Design review of the part built by this model. Coordinates are the model's own, in mm. A direction names the side the tool comes from. Coordinates: 2 decimals unless noted, no trailing zeros. Loops run counter-clockwise (first coordinate to the right, second up) from the corner with the lowest first, then second, coordinate; pieces in that order, holes last. Notation, with made-up numbers: M 43.25,59.5 L 97.25,59.5 A19 cw 97.25,71.5 Z; hole C 13.25,7.25 d1. An arc over 180 degrees is marked long. Write item = value, one per line. Start each with the question number.
from build123d import *

# Parameters (mm, degrees)
SKETCH1_W                = 50
SKETCH1_H                = 25
SKETCH1_R                = 1.3
SKETCH1_R_2              = 4.5
BOSS_EXTRUDE1_DEPTH      = 2.5
SKETCH2_W                = 50
SKETCH2_H                = 12
BOSS_EXTRUDE2_DEPTH      = 3
SKETCH3_W                = 50
SKETCH3_H                = 28
BOSS_EXTRUDE3_DEPTH      = 3
SKETCH4_R                = 1.3
CUT_EXTRUDE1_DEPTH       = 16
SKETCH5_W                = 53
SKETCH5_H                = 32.5
SKETCH5_R                = 1.6
SKETCH5_W_2              = 42
SKETCH5_H_2              = 21.5
BOSS_EXTRUDE4_DEPTH      = 4
SKETCH7_R                = 8
CUT_EXTRUDE2_DEPTH       = 5
SKETCH8_W                = 24.55
SKETCH8_H                = 21.5
CUT_EXTRUDE3_DEPTH       = 3.8
BOSS_EXTRUDE6_DEPTH      = 22.95
BOSS_EXTRUDE7_DEPTH      = 2
SKETCH11_R               = 1.6
CUT_EXTRUDE4_DEPTH       = 1.2
SKETCH12_W               = 7
SKETCH12_H               = 21
SKETCH12_R               = 1.6
BOSS_EXTRUDE8_DEPTH      = 7.8
SKETCH13_W               = 0.7
SKETCH13_H               = 5
SKETCH13_H_2             = 4
CUT_EXTRUDE5_DEPTH       = 51
CUT_EXTRUDE5_DEPTH_BACK  = 25.95
SKETCH14_W               = 28
SKETCH14_H               = 10
CUT_EXTRUDE6_DEPTH       = 1
CUT_EXTRUDE6_DEPTH_BACK  = 75.95
SKETCH16_R               = 3
CUT_EXTRUDE8_DEPTH       = 3
SKETCH15_R               = 1.6
CUT_EXTRUDE9_DEPTH       = 5
SKETCH17_W               = 16.3
SKETCH17_H               = 5
CUT_EXTRUDE10_DEPTH      = 3.2
SKETCH18_R               = 1.45
CUT_EXTRUDE11_DEPTH      = 5
SKETCH19_R               = 1.6
CUT_EXTRUDE12_DEPTH      = 1.0000001
CUT_EXTRUDE12_DEPTH_BACK = 10
SKETCH20_W               = 17.95
SKETCH20_H               = 5
CUT_EXTRUDE14_DEPTH      = 1
CUT_EXTRUDE14_DEPTH_BACK = 32.8
SKETCH21_W               = 16.3
SKETCH21_H               = 5
SKETCH21_R               = 1.45
BOSS_EXTRUDE11_DEPTH     = 2
SKETCH22_W               = 55
SKETCH22_H               = 5
BOSS_EXTRUDE12_DEPTH     = 25
SKETCH23_R               = 10.5
BOSS_EXTRUDE13_DEPTH     = 2
SKETCH24_R               = 1.3
SKETCH24_R_2             = 0.75
CUT_EXTRUDE16_DEPTH      = 7
SKETCH25_R               = 2.5
SKETCH25_R_2             = 1.3
CUT_EXTRUDE17_DEPTH      = 4


with BuildPart() as part:
    # Sketch1 → Boss-Extrude1 (new body, symmetric)
    with BuildSketch(Plane(origin=(0, 0, 0), x_dir=(1, 0, 0), z_dir=(0, 1, 0))):
        Rectangle(SKETCH1_W, SKETCH1_H)
        with Locations((-11.25, 0)):
            Circle(SKETCH1_R, mode=Mode.SUBTRACT)
        with Locations((11.25, 0)):
            Circle(SKETCH1_R_2, mode=Mode.SUBTRACT)
    extrude(amount=BOSS_EXTRUDE1_DEPTH, both=True)

    # Sketch2 → Boss-Extrude2 (add)
    with BuildSketch(Plane.XY.offset(12.5)):
        with Locations((0, 3.5)):
            Rectangle(SKETCH2_W, SKETCH2_H)
    extrude(amount=BOSS_EXTRUDE2_DEPTH)

    # Sketch3 → Boss-Extrude3 (add)
    with BuildSketch(Plane(origin=(0, 9.5, 0), x_dir=(1, 0, 0), z_dir=(0, 1, 0))):
        with Locations((0, -1.5)):
            Rectangle(SKETCH3_W, SKETCH3_H)
    extrude(amount=BOSS_EXTRUDE3_DEPTH)

    # Sketch4 → Cut-Extrude1 (cut, through all)
    with BuildSketch(Plane(origin=(0, 12.5, 0), x_dir=(1, 0, 0), z_dir=(0, 1, 0))):
        with Locations((11.25, 0)):
            Circle(SKETCH4_R)
        with Locations((-11.25, 0)):
            Circle(SKETCH4_R)
    extrude(amount=-CUT_EXTRUDE1_DEPTH, mode=Mode.SUBTRACT)

    # Sketch5 → Boss-Extrude4 (add)
    with BuildSketch(Plane.XZ.offset(2.5)):
        with Locations((21.45, -0.05)):
            Rectangle(SKETCH5_W, SKETCH5_H)
        with Locations((45.75, -5)):
            Circle(SKETCH5_R, mode=Mode.SUBTRACT)
        with Locations((45.75, 4.9)):
            Circle(SKETCH5_R, mode=Mode.SUBTRACT)
        with Locations((-2.85, 4.9)):
            Circle(SKETCH5_R, mode=Mode.SUBTRACT)
        with Locations((-2.85, -5)):
            Circle(SKETCH5_R, mode=Mode.SUBTRACT)
        with Locations((21.45, -0.05)):
            Rectangle(SKETCH5_W_2, SKETCH5_H_2, mode=Mode.SUBTRACT)
    extrude(amount=BOSS_EXTRUDE4_DEPTH)

    # Sketch7 → Cut-Extrude2 (cut)
    with BuildSketch(Plane.XZ.offset(2.5)):
        with Locations((11.25, 0)):
            Circle(SKETCH7_R)
    extrude(amount=-CUT_EXTRUDE2_DEPTH, mode=Mode.SUBTRACT)

    # Sketch8 → Cut-Extrude3 (cut)
    with BuildSketch(Plane.XZ.offset(2.5)):
        with Locations((12.725, -0.05)):
            Rectangle(SKETCH8_W, SKETCH8_H)
    extrude(amount=-CUT_EXTRUDE3_DEPTH, mode=Mode.SUBTRACT)

    # Sketch9 → Boss-Extrude6 (add)
    with BuildSketch(Plane(origin=(25, 0, 0), x_dir=(0, 0, -1), z_dir=(1, 0, 0))):
        Polygon((12.5, 2.5), (-16.2, 2.5), (-16.2, -2.5), (-10.7, -2.5), (-10.7, 1.3), (10.8, 1.3), (10.8, -2.5), (12.5, -2.5), align=None)
    extrude(amount=BOSS_EXTRUDE6_DEPTH)

    # Sketch10 → Boss-Extrude7 (add)
    with BuildSketch(Plane(origin=(47.95, 0, 0), x_dir=(0, 0, -1), z_dir=(1, 0, 0))):
        Polygon((16.3, -2.5), (12.5, -2.5), (12.5, 2.5), (-16.2, 2.5), (-16.2, -6.5), (16.3, -6.5), align=None)
    extrude(amount=BOSS_EXTRUDE7_DEPTH)

    # Sketch11 → Cut-Extrude4 (cut)
    with BuildSketch(Plane.XZ.offset(-1.3)):
        with Locations((-2.85, 4.9)):
            Circle(SKETCH11_R)
        with Locations((-2.85, -5)):
            Circle(SKETCH11_R)
        with Locations((45.75, 4.9)):
            Circle(SKETCH11_R)
        with Locations((45.75, -5)):
            Circle(SKETCH11_R)
    extrude(amount=-CUT_EXTRUDE4_DEPTH, mode=Mode.SUBTRACT)

    # Sketch12 → Boss-Extrude8 (add)
    with BuildSketch(Plane.XZ.offset(-1.3)):
        with Locations((46.45, 0.2)):
            Rectangle(SKETCH12_W, SKETCH12_H)
        with Locations((45.75, 4.9)):
            Circle(SKETCH12_R, mode=Mode.SUBTRACT)
        with Locations((45.75, -5)):
            Circle(SKETCH12_R, mode=Mode.SUBTRACT)
    extrude(amount=BOSS_EXTRUDE8_DEPTH)

    # Sketch13 → Cut-Extrude5 (cut, two sides)
    with BuildSketch(Plane.ZY.offset(-25)) as cut_extrude5_sk:
        with Locations((15.85, 0)):
            Rectangle(SKETCH13_W, SKETCH13_H)
        with Locations((15.85, -4.5)):
            Rectangle(SKETCH13_W, SKETCH13_H_2)
    extrude(amount=CUT_EXTRUDE5_DEPTH, mode=Mode.SUBTRACT)
    extrude(cut_extrude5_sk.sketch, amount=-CUT_EXTRUDE5_DEPTH_BACK, mode=Mode.SUBTRACT)

    # Sketch14 → Cut-Extrude6 (cut, two sides)
    with BuildSketch(Plane.ZY.offset(25)) as cut_extrude6_sk:
        with Locations((1.5, 7.5)):
            Rectangle(SKETCH14_W, SKETCH14_H)
    extrude(amount=CUT_EXTRUDE6_DEPTH, mode=Mode.SUBTRACT)
    extrude(cut_extrude6_sk.sketch, amount=-CUT_EXTRUDE6_DEPTH_BACK, mode=Mode.SUBTRACT)

    # Sketch16 → Cut-Extrude8 (cut)
    with BuildSketch(Plane(origin=(0, 2.5, 0), x_dir=(1, 0, 0), z_dir=(0, 1, 0))):
        with Locations((-2.85, 5)):
            Circle(SKETCH16_R)
        with Locations((-2.85, -4.9)):
            Circle(SKETCH16_R)
        with Locations((45.75, 5)):
            Circle(SKETCH16_R)
        with Locations((45.75, -4.9)):
            Circle(SKETCH16_R)
    extrude(amount=-CUT_EXTRUDE8_DEPTH, mode=Mode.SUBTRACT)

    # Sketch15 → Cut-Extrude9 (cut)
    with BuildSketch(Plane(origin=(0, 2.5, 0), x_dir=(1, 0, 0), z_dir=(0, 1, 0))):
        with Locations((-2.85, 5)):
            Circle(SKETCH15_R)
        with Locations((-2.85, -4.9)):
            Circle(SKETCH15_R)
    extrude(amount=-CUT_EXTRUDE9_DEPTH, mode=Mode.SUBTRACT)

    # Sketch17 → Cut-Extrude10 (cut)
    with BuildSketch(Plane.XY.offset(15.5)):
        with Locations((8.9, 0)):
            Rectangle(SKETCH17_W, SKETCH17_H)
        with Locations((31, 0)):
            Rectangle(SKETCH17_W, SKETCH17_H)
    extrude(amount=-CUT_EXTRUDE10_DEPTH, mode=Mode.SUBTRACT)

    # Sketch18 → Cut-Extrude11 (cut)
    with BuildSketch(Plane.XY.offset(12.3)):
        with Locations((8.95, 0)):
            Circle(SKETCH18_R)
        with Locations((30.95, 0)):
            Circle(SKETCH18_R)
    extrude(amount=-CUT_EXTRUDE11_DEPTH, mode=Mode.SUBTRACT)

    # Sketch19 → Cut-Extrude12 (cut, two sides)
    with BuildSketch(Plane(origin=(0, 2.5, 0), x_dir=(1, 0, 0), z_dir=(0, 1, 0))) as cut_extrude12_sk:
        with Locations((33.75, 0)):
            Circle(SKETCH19_R)
    extrude(amount=CUT_EXTRUDE12_DEPTH, mode=Mode.SUBTRACT)
    extrude(cut_extrude12_sk.sketch, amount=-CUT_EXTRUDE12_DEPTH_BACK, mode=Mode.SUBTRACT)

    # Sketch20 → Cut-Extrude14 (cut, two sides)
    with BuildSketch(Plane.XY.offset(15.5)) as cut_extrude14_sk:
        with Locations((-16.025, 0)):
            Rectangle(SKETCH20_W, SKETCH20_H)
    extrude(amount=CUT_EXTRUDE14_DEPTH, mode=Mode.SUBTRACT)
    extrude(cut_extrude14_sk.sketch, amount=-CUT_EXTRUDE14_DEPTH_BACK, mode=Mode.SUBTRACT)

    # Sketch21 → Boss-Extrude11 (add)
    with BuildSketch(Plane.XY.offset(15.5)):
        with Locations((8.9, 0)):
            Rectangle(SKETCH21_W, SKETCH21_H)
        with Locations((8.95, 0)):
            Circle(SKETCH21_R, mode=Mode.SUBTRACT)
        Polygon((0.75, -2.5), (0.75, 2.5), (-7.05, 2.5), (-7.05, -2.5), (-5.05, -2.5), (-5.05, -6.5), (49.95, -6.5), (49.95, 2.5), (39.15, 2.5), (39.15, -2.5), (22.85, -2.5), (22.85, 2.5), (17.05, 2.5), (17.05, -2.5), align=None)
        with Locations((31, 0)):
            Rectangle(SKETCH21_W, SKETCH21_H)
        with Locations((30.95, 0)):
            Circle(SKETCH21_R, mode=Mode.SUBTRACT)
    extrude(amount=BOSS_EXTRUDE11_DEPTH)

    # Sketch22 → Boss-Extrude12 (add)
    with BuildSketch(Plane.XZ.offset(6.5)):
        with Locations((22.45, 15)):
            Rectangle(SKETCH22_W, SKETCH22_H)
    extrude(amount=BOSS_EXTRUDE12_DEPTH)

    # Sketch23 → Boss-Extrude13 (add)
    with BuildSketch(Plane.XY.offset(17.5)):
        with Locations((22.45, -19.5)):
            Circle(SKETCH23_R)
    extrude(amount=BOSS_EXTRUDE13_DEPTH)

    # Sketch24 → Cut-Extrude16 (cut)
    with BuildSketch(Plane.XY.offset(19.5)):
        with Locations((22.45, -19.5)):
            Circle(SKETCH24_R)
        with Locations((22.45, -11.8)):
            Circle(SKETCH24_R_2)
        with Locations((22.45, -27.2)):
            Circle(SKETCH24_R_2)
    extrude(amount=-CUT_EXTRUDE16_DEPTH, mode=Mode.SUBTRACT)

    # Sketch25 → Cut-Extrude17 (cut)
    with BuildSketch(Plane(origin=(0, 0, 12.5), x_dir=(-1, 0, 0), z_dir=(0, 0, -1))):
        with Locations((-22.45, -19.5)):
            Circle(SKETCH25_R)
        with Locations((-22.45, -19.5)):
            Circle(SKETCH25_R_2, mode=Mode.SUBTRACT)
    extrude(amount=-CUT_EXTRUDE17_DEPTH, mode=Mode.SUBTRACT)


solid = part.part
Q1. For faces 5 (the face through (31, -2.5, 14)), 6 (the face through (22, -2.5, -14)), 7 (the face through (11.96, -19.04, 18.49)), 8 (the face through (22, -16, 12.5)), 9 (the face through (21, -21, 16.5)), list the 3-axis set-ups (+Z, -Z, +X, -X, +Y, -Y) from which the entire face can be reached by the end or side of a thin tool; tool diameter is ignored.
Q2. Add section B-B on z = 0. State the section outline as (x, y) points.
Q3. Add section C-C on x = -2.85. State the section outline as (y, z) points.
Q4. To check wall thickness, follow line 1 (X direction, y = 1.65, z = 0); line 2 (Z direction, x = -2.85, y = 1.1); line 3 (Z direction, x = -2.85, y = -4.7). State the ranges of each line that lie inside material, in increasing order. Write a range as from..to.
Q5. Mouldability with a two-part tool opening along Z and no side actions: class faces 1 (the face through (44.57, -3.46, -3.92)), 2 (the face through (24, 1.3, 0)), 3 (the face through (10, -1, 16)), 4 (the face through (22, -5, -16.3)) as released by +Z, released by -Z, zero draft, split by the parting line, or undercut.
Q6. Clearance check with flat-ended pins moving along their axes: P1, Ø1.7, axis at x = 45.5, z = 6, coming from the +Y side; P2, Ø7.5, axis at x = 17.5, y = -24.5, coming from the -Z side; P3, Ø3, axis at x = 17, z = -14.5, coming from the +Y side. State where each tip first meets the part, or that it passes through.
Q7. Add section D-D on x = 11.25. State the section outline as (y, z) points.
Q8. Add section A-A on x = 45.75. State the section outline as (y, z) points.
Values follow:
q1.face_5 = +Y
q1.face_6 = -Z, +X, -X, +Y
q1.face_7 = +Z
q1.face_8 = -Z, +X, -X, -Y
q1.face_9 = -Z
q2.outline = M -7.05,-2.5 L -5.05,-2.5 L -5.05,-6.5 L 0.45,-6.5 L 0.45,1.3 L 3.25,1.3 L 3.25,2.5 L -7.05,2.5 Z; M 19.25,1.3 L 32.15,1.3 L 32.15,2.5 L 19.25,2.5 Z; M 35.35,1.3 L 42.95,1.3 L 42.95,-2.5 L 42.45,-2.5 L 42.45,-6.5 L 49.95,-6.5 L 49.95,2.5 L 35.35,2.5 Z
q3.outline = M -31.5,12.5 L -6.5,12.5 L -6.5,6.5 L -0.5,6.5 L -0.5,7.9 L 2.5,7.9 L 2.5,17.5 L -31.5,17.5 Z; M -6.5,-16.3 L -2.5,-16.3 L -2.5,-12.5 L 2.5,-12.5 L 2.5,-8 L -0.5,-8 L -0.5,-6.6 L -6.5,-6.6 Z; M -6.5,-3.4 L -0.5,-3.4 L -0.5,-2 L 2.5,-2 L 2.5,1.9 L -0.5,1.9 L -0.5,3.3 L -6.5,3.3 Z
q4.line_1 = -7.05..3.25, 19.25..32.15, 35.35..49.95
q4.line_2 = -12.5..-8, -2..1.9, 7.9..17.5
q4.line_3 = -16.3..-6.6, -3.4..3.3, 6.5..17.5
q5.face_1 = undercut
q5.face_2 = undercut
q5.face_3 = zero draft
q5.face_4 = released by -Z
q6.P1 = -0.5
q6.P2 = 12.5
q6.P3 = -2.5
q7.outline = M -31.5,12.5 L -6.5,12.5 L -6.5,10.7 L 1.3,10.7 L 1.3,8 L 2.5,8 L 2.5,12.3 L -2.5,12.3 L -2.5,15.5 L 2.5,15.5 L 2.5,17.5 L -31.5,17.5 Z; M -6.5,-16.3 L -2.5,-16.3 L -2.5,-12.5 L 2.5,-12.5 L 2.5,-8 L 1.3,-8 L 1.3,-10.8 L -6.5,-10.8 Z
q8.outline = M -31.5,12.5 L -6.5,12.5 L -6.5,6.5 L -0.5,6.5 L -0.5,7.9 L 2.5,7.9 L 2.5,17.5 L -31.5,17.5 Z; M -6.5,-16.3 L -2.5,-16.3 L -2.5,-12.5 L 2.5,-12.5 L 2.5,-8 L -0.5,-8 L -0.5,-6.6 L -6.5,-6.6 Z; M -6.5,-3.4 L -0.5,-3.4 L -0.5,-2 L 2.5,-2 L 2.5,1.9 L -0.5,1.9 L -0.5,3.3 L -6.5,3.3 Z; hole M -2.5,-10.8 L 1.3,-10.8 L 1.3,-10.3 L -2.5,-10.3 Z
